from build123d import *

# Parameters (mm, degrees)
F0_R      = 30
F0_R_2    = 27
F1_DEPTH  = 4
F4_R      = 30
F3_R      = 23
F7_R      = 20
F6_R      = 27
F9_R      = 22.403667
F9_R_2    = 12.693191
F10_DEPTH = 2
F11_R     = 35
F11_R_2   = 27
F12_DEPTH = 3
F13_R     = 1.5
F14_DEPTH = 25


with BuildPart() as f1:
    # F0 (on Front) → F1 (new body)
    with BuildSketch(Plane.XZ):
        Circle(F0_R)
        Circle(F0_R_2, mode=Mode.SUBTRACT)
    extrude(amount=F1_DEPTH)

    # F4 (on face) → F5 section 0
    with BuildSketch(Plane.XZ.offset(4)):
        Circle(F4_R)
    # F3 (on offset) → F5 section 1
    with BuildSketch(Plane.XZ.offset(38)):
        Circle(F3_R)
    loft()

    # F7 (on face) → F8 section 0
    with BuildSketch(Plane.XZ.offset(38)):
        Circle(F7_R)
    # F6 (on face) → F8 section 1
    with BuildSketch(Plane(origin=(0, -4, 0), x_dir=(-1, 0, 0), z_dir=(0, 1, 0))):
        Circle(F6_R)
    loft(mode=Mode.SUBTRACT)

    # F9 (on face) → F10 (join)
    with BuildSketch(Plane.XZ.offset(38)):
        Circle(F9_R)
        Circle(F9_R_2, mode=Mode.SUBTRACT)
    extrude(amount=-F10_DEPTH)

    # F11 (on face) → F12 (join)
    with BuildSketch(Plane(origin=(0, 0, 0), x_dir=(-1, 0, 0), z_dir=(0, 1, 0))):
        Circle(F11_R)
        Circle(F11_R_2, mode=Mode.SUBTRACT)
    extrude(amount=F12_DEPTH)

    # F13 (on face) → F14 (cut)
    with BuildSketch(Plane(origin=(0, 3, 0), x_dir=(-1, 0, 0), z_dir=(0, 1, 0))):
        with Locations((-4.877913, 31.626033)):
            Circle(F13_R)
        with Locations((24.949992, 20.037413)):
            Circle(F13_R)
        with Locations((29.827904, -11.58862)):
            Circle(F13_R)
        with Locations((4.877913, -31.626033)):
            Circle(F13_R)
        with Locations((-24.949992, -20.037413)):
            Circle(F13_R)
        with Locations((-29.827904, 11.58862)):
            Circle(F13_R)
    extrude(amount=-F14_DEPTH, mode=Mode.SUBTRACT)


solid = f1.part
The listing builds one solid part. Answer for the finished solid, in the listing's coordinates (mm). A direction names the side the tool comes from. Give positions to 0.01 mm unless a question says otherwise; leave off trailing zeros. Order: outer loops, then holes, each group sorted by start corner. A loop starts at its lowest first (then second) coordinate and runs counter-clockwise, first axis right, second up. Notation, with made-up numbers: (27.5, -5.75) - (72.5, -5.75) arc R22 ccw to (72.5, 17.25) - close; hole circle Ø6 at (-9.75, 62.25). An arc over 180 degrees is marked (long way). Answer as CSV lines item,"result".
Q1. A cutting plane is placed at B-B, the plane y = -26. Determine the outline of the cut face in (x, z), and give its area (3 significant figures).
Answer key:
outline,"circle Ø50.94 at (0, 0); hole circle Ø44.94 at (0, 0)"
area,"452 mm^2"
Q2. Each of these flat-tipped pins is pushed along its axis until it touches: pin 1 Ø2.5 at (x, z) = (4.88, 31.63) entering from -Y; pin 2 Ø6 at (x, z) = (-25, 4.5) entering from +Y; pin 3 Ø3 at (y, z) = (-8.5, -25.5) entering from +X; pin 4 Ø6 at (x, y) = (-5, -19.5) entering from +Z. Where does it stop, or does it pass through?
Answer key:
pin 1,"passes through"
pin 2,"stops at y = 3"
pin 3,"stops at x = 16.48"
pin 4,"stops at z = 27.12"
Q3. A cutting plane is placed at A-A, the plane x = 0. Determine the outline of the cut face in (y, z), and give its area (3 significant figures).
Answer key:
outline,"(-38, -23) - (-4, -30) - (0, -30) - (0, -35) - (3, -35) - (3, -27) - (-4, -27) - (-36, -20.41) - (-36, -12.69) - (-38, -12.69) - close; (-38, 12.69) - (-36, 12.69) - (-36, 20.41) - (-4, 27) - (3, 27) - (3, 35) - (0, 35) - (0, 30) - (-4, 30) - (-38, 23) - close"
area,"306 mm^2"
Q4. Determine the mould class of faces 4 (the face through (10, -38, -10)), 5 (the face through (28, 1, -21)), 6 (the face through (3.45, 1.52, 32.08)) for opening direction Z: pulls with the +Z half, pulls with the -Z half, needs draft (parallel to the pull), parting line crosses it, or undercut.
Answer key:
face 4,"needs draft"
face 5,"parting line crosses it"
face 6,"undercut"
Q5. Straight lines are drawn through the part: L1, parallel to Z at x = 0, y = -2; L2, parallel to Y at x = 19, z = -25.5; L3, parallel to Z at x = 15.5, y = -7.5. For each, find the intervals that lie inside material, in ascending order.
Answer key:
L1,"z = -30 to -27, 27 to 30"
L2,"y = 0 to 3"
L3,"z = -24.84 to -21.22, 21.22 to 24.84"
Q6. Which of the six approach directions +Z, -Z, +X, -X, +Y, -Y give full straight-line access (tool end or side, diameter ignored) to faces 1 (the face through (8.8, -36, 9.4)), 2 (the face through (10.5, 0, -28.4)), 3 (the face through (-31.26, 1.52, -11.14))?
Answer key:
face 1,"+Y"
face 2,"-Y"
face 3,"+Y, -Y"
Q7. A cutting plane is placed at C-C, the plane y = -11.5. Determine the outline of the cut face in (x, z).
Answer key:
outline,"circle Ø56.91 at (0, 0); hole circle Ø50.91 at (0, 0)"
